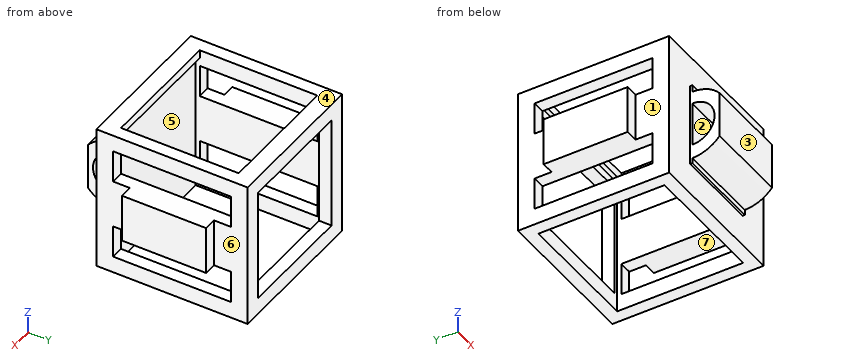
from build123d import *

# Parameters (mm, degrees)
SKETCH1_W               = 36
SKETCH1_H               = 36
BOSS_EXTRUDE1_DEPTH     = 17.5
SKETCH2_W               = 30
SKETCH2_H               = 30
CUT_EXTRUDE1_DEPTH      = 15.5
CUT_EXTRUDE1_DEPTH_BACK = 18.5
SKETCH3_W               = 30
SKETCH3_H               = 28
CUT_EXTRUDE3_DEPTH      = 36
SKETCH5_W               = 20
SKETCH5_H               = 20
BOSS_EXTRUDE2_DEPTH     = 7
CUT_EXTRUDE4_DEPTH      = 29
SKETCH7_W               = 11.5
SKETCH7_H               = 20
BOSS_EXTRUDE3_DEPTH     = 3
CUT_EXTRUDE5_DEPTH      = 32
CUT_EXTRUDE6_REACH      = 45
SKETCH10_W              = 28
SKETCH10_H              = 27
SKETCH11_W              = 7.75
SKETCH11_H              = 28
CUT_EXTRUDE7_DEPTH      = 40


with BuildPart() as part:
    # Sketch1 → Boss-Extrude1 (new body, symmetric)
    with BuildSketch(Plane.XY):
        Rectangle(SKETCH1_W, SKETCH1_H)
    extrude(amount=BOSS_EXTRUDE1_DEPTH, both=True)

    # Sketch2 → Cut-Extrude1 (cut, two sides)
    with BuildSketch(Plane.XY) as cut_extrude1_sk:
        Rectangle(SKETCH2_W, SKETCH2_H)
    extrude(amount=CUT_EXTRUDE1_DEPTH, mode=Mode.SUBTRACT)
    extrude(cut_extrude1_sk.sketch, amount=-CUT_EXTRUDE1_DEPTH_BACK, mode=Mode.SUBTRACT)

    # Sketch3 → Cut-Extrude3 (cut, through all)
    with BuildSketch(Plane.XY.offset(17.5)):
        Rectangle(SKETCH3_W, SKETCH3_H)
    extrude(amount=-CUT_EXTRUDE3_DEPTH, mode=Mode.SUBTRACT)

    # Sketch5 → Boss-Extrude2 (add)
    with BuildSketch(Plane(origin=(0, -18, 0), x_dir=(-1, 0, 0), z_dir=(0, -1, 0))):
        Rectangle(SKETCH5_W, SKETCH5_H)
    extrude(amount=BOSS_EXTRUDE2_DEPTH)

    # Sketch6 → Cut-Extrude4 (cut, through all)
    with BuildSketch(Plane(origin=(10, 0, 0), x_dir=(0, 0, -1), z_dir=(1, 0, 0))):
        with BuildLine():
            Line((-5.3, -18.5), (5.3, -18.5))
            ThreePointArc((5.3, -18.5), (0, -23.8), (-5.3, -18.5))
        make_face()
    extrude(amount=-CUT_EXTRUDE4_DEPTH, mode=Mode.SUBTRACT)

    # Sketch7 → Boss-Extrude3 (add)
    with BuildSketch(Plane(origin=(18, 0, 0), x_dir=(0, 0, -1), z_dir=(1, 0, 0))):
        Rectangle(SKETCH7_W, SKETCH7_H)
    boss_extrude3 = extrude(amount=BOSS_EXTRUDE3_DEPTH)

    # Mirror1: Boss-Extrude3 across plane
    add(boss_extrude3.mirror(Plane(origin=(0, 0, 0), x_dir=(0, 0, 1), z_dir=(1, 0, 0))))

    # Sketch9 → Cut-Extrude5 (cut, through all)
    with BuildSketch(Plane(origin=(10, 0, 0), x_dir=(0, 0, -1), z_dir=(1, 0, 0))):
        with BuildLine():
            Line((-8.3, -18.5), (-10, -18.5))
            Line((-10, -18.5), (-10, -28.666019684))
            Line((-10, -28.666019684), (10, -28.666019684))
            Line((10, -28.666019684), (10, -18.5))
            Line((10, -18.5), (8.709331347, -18.5))
            ThreePointArc((8.709331347, -18.5), (0.204665673, -27.004665673), (-8.3, -18.5))
        make_face()
    extrude(amount=-CUT_EXTRUDE5_DEPTH, mode=Mode.SUBTRACT)

    # Sketch10 → Cut-Extrude6 (cut, up to next)
    with BuildSketch(Plane(origin=(0, 18, 0), x_dir=(1, 0, 0), z_dir=(0, 1, 0)), mode=Mode.PRIVATE) as cut_extrude6_sk1:
        Rectangle(SKETCH10_W, SKETCH10_H)
    cut_extrude6_tool1 = extrude(cut_extrude6_sk1.sketch, amount=-CUT_EXTRUDE6_REACH, mode=Mode.PRIVATE) & part.part
    add(cut_extrude6_tool1.solids().sort_by_distance((0, 18, 0))[0], mode=Mode.SUBTRACT)

    # Sketch11 → Cut-Extrude7 (cut, through all)
    with BuildSketch(Plane(origin=(18, 0, 0), x_dir=(0, 0, -1), z_dir=(1, 0, 0))):
        with Locations((-9.625, 0)):
            Rectangle(SKETCH11_W, SKETCH11_H)
        with Locations((9.625, 0)):
            Rectangle(SKETCH11_W, SKETCH11_H)
    extrude(amount=-CUT_EXTRUDE7_DEPTH, mode=Mode.SUBTRACT)


solid = part.part
Geometry: final body of the model. Coordinates: model frame, mm. Face numbers are marked on the shaded views. A direction names the side the tool comes from. Round coordinates to 2 decimals unless told otherwise and drop trailing zeros. Loops run counter-clockwise (first coordinate to the right, second up) from the corner with the lowest first, then second, coordinate; pieces in that order, holes last.
Q1. Section D-D on z = 0. Return loops of the section in (x, y).
Q2. Section B-B on x = 1. Return loops of the section in (y, z), plus the area to 3 significant figures.
Q3. Material intervals for L1, parallel to Z at x = -16, y = -7; L2, parallel to X at y = -12, z = 15, sorted ascending.
Q4. Pin query (flat end, axial travel): P1, Ø15, axis at x = 6, z = 3.5, coming from the +Y side; P2, Ø1.5, axis at x = 16, z = -10.5, coming from the -Y side; P3, Ø0.9, axis at y = 16, z = 2.5, coming from the +X side. Return the tip coordinate at first contact, or that it passes through.
Q5. Section A-A on y = 13. Return loops of the section in (x, z).
Q6. Section C-C on z = 11.5. Return loops of the section in (x, y), plus the area to 3 significant figures.
Q7. Access query for the marked faces 4, 5, 6 and 7. Directions: +Z, -Z, +X, -X, +Y, -Y. A direction counts if a zero-diameter tool reaches every point of the face in a straight line with its end or side. Return the directions, or none.
Q8. Pull-direction query (Y, two-part tool) for the marked faces 1, 2 and 3; classes: released by +Y, released by -Y, zero draft, split by the parting line, or undercut.
Evaluation:
1. outline: (-21, -10) - (-18, -10) - (-18, -18) - (-10, -18) - (-10, -18.5) - (10, -18.5) - (10, -18) - (18, -18) - (18, -10) - (21, -10) - (21, 10) - (18, 10) - (18, 18) - (14, 18) - (14, 15) - (15, 15) - (15, -15) - (-15, -15) - (-15, 15) - (-14, 15) - (-14, 18) - (-18, 18) - (-18, 10) - (-21, 10) - close; (-10, -25) - (10, -25) - (10, -23.8) - (-10, -23.8) - close
2. outline: (-25, -5.69) arc R8.5 ccw to (-18.5, -8.71) - (-18.5, -10) - (-18, -10) - (-18, -17.5) - (-15, -17.5) - (-15, 15.5) - (-14, 15.5) - (-14, 17.5) - (-18, 17.5) - (-18, 10) - (-18.5, 10) - (-18.5, 8.3) arc R8.5 ccw to (-25, 5.28) - close; (14, 15.5) - (15, 15.5) - (15, 13.5) - (18, 13.5) - (18, 17.5) - (14, 17.5) - close; (15, -17.5) - (18, -17.5) - (18, -13.5) - (15, -13.5) - close; hole (-18.5, -5.3) - (-18.5, 5.3) arc R5.3 ccw to start
2. area: 197 mm2
3. L1: z = -17.5 to -13.5, -5.75 to 5.75, 13.5 to 17.5
3. L2: x = -18 to -15, 15 to 18
4. P1: stops at y = -15
4. P2: stops at y = -18
4. P3: stops at x = 18
5. outline: (-18, -17.5) - (-15, -17.5) - (-15, -13.5) - (-18, -13.5) - close; (-18, -5.75) - (-15, -5.75) - (-15, 5.75) - (-18, 5.75) - close; (-18, 13.5) - (-15, 13.5) - (-15, 17.5) - (-18, 17.5) - close; (15, -17.5) - (18, -17.5) - (18, -13.5) - (15, -13.5) - close; (15, -5.75) - (18, -5.75) - (18, 5.75) - (15, 5.75) - close; (15, 13.5) - (18, 13.5) - (18, 17.5) - (15, 17.5) - close
6. outline: (-18, -18) - (18, -18) - (18, -14) - (15, -14) - (15, -15) - (-15, -15) - (-15, -14) - (-18, -14) - close; (-18, 14) - (-15, 14) - (-15, 15) - (-14, 15) - (-14, 18) - (-18, 18) - close; (14, 15) - (15, 15) - (15, 14) - (18, 14) - (18, 18) - (14, 18) - close
6. area: 144 mm2
7. face 4: +Z, +X, -X, +Y, -Y
7. face 5: -Z
7. face 6: +X
7. face 7: +X, -X
8. face 1: zero draft
8. face 2: undercut
8. face 3: released by -Y
